Geometry: see drawing. Coordinates: mm, zero at the bounding-box minimum. A direction names the side the tool comes from. Give positions to 0.01 mm unless a question says otherwise; leave off trailing zeros. Order: outer loops, then holes, each group sorted by start corner. A loop starts at its lowest first (then second) coordinate and runs counter-clockwise, first axis right, second up. Notation, with made-up numbers: M 2,-24 L 46,-24 A21 cw 46,-11 Z; hole C 13,9.5 d7. An arc over 180 degrees is marked long. Answer as a JSON object with one key per item and string values. Group by question number.
1. Section query A-A (y = 69.85). Count the separate pieces of the cut face and the enclosed holes in it, plus the area to 3 significant figures.
2. Pull-direction query (Y, two-part tool) for the marked faces 1, 2, 3 and 4; classes: +Y half, -Y half, draft (parallel to the pull), parting line (faces both ways), or undercut.
3. Set-up query: the marked faces 5, 6, 7, 8 and 9. Return all of +Z, -Z, +X, -X, +Y, -Y with unobstructed straight access to the full face (end or side cutting, diameter ignored); none if empty.
4. Section query D-D (x = 406.5). Output: boundary loops of the cut face in (y, z), plus the area to 3 significant figures.
5. Pin query (flat end, axial travel): P1, Ø11.5, axis at x = 37.5, z = 11, coming from the +Y side; P2, Ø19, axis at y = 105.5, z = 17, coming from the -X side; P3, Ø3, axis at y = 22.5, z = 32.5, coming from the +X side; P4, Ø7.5, axis at x = 44.45, z = 19.05, coming from the -Y side. Return the tip coordinate at first contact, or that it passes through.
6. Section query C-C (x = 44.45). Output: boundary loops of the cut face in (y, z), plus the area to 3 significant figures.
7. Section query B-B (z = 19.05). Output: boundary loops of the cut face in (x, y).
8. Material intervals for L1, parallel to X at y = 71, z = 20 (1 decimal); L2, parallel to Z at x = 527, y = 81; L3, parallel to X at y = 19, z = 28.5, sorted ascending. Write a range as [from, to].
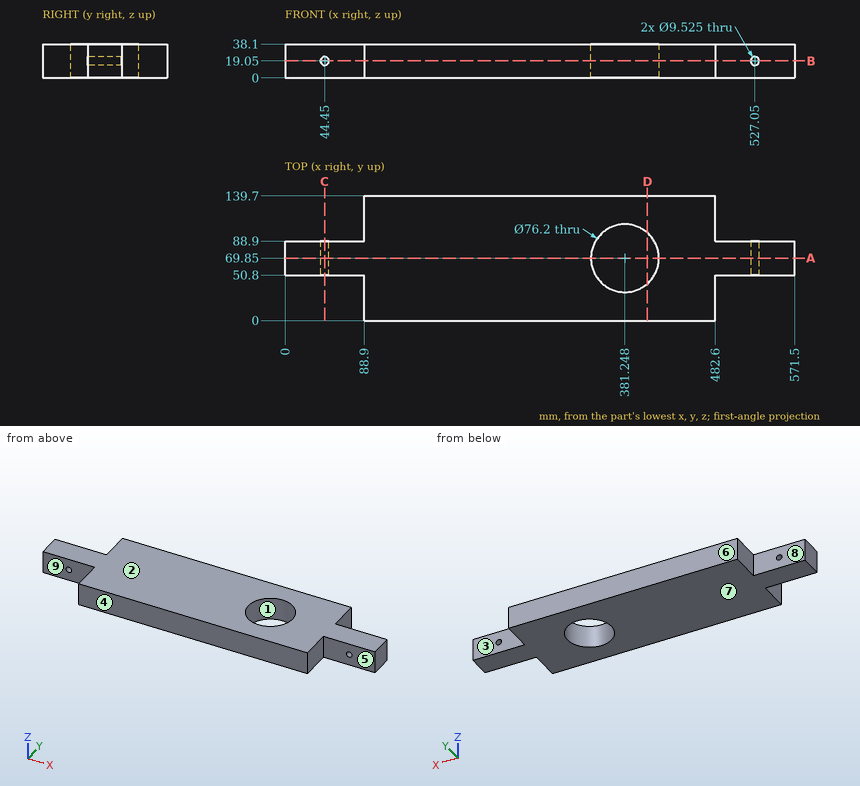
Answer sheet:
{
 "1": {"separate pieces": "2", "enclosed holes": "2", "area": "18,700 mm^2"},
 "2": {"face 1": "undercut", "face 2": "draft", "face 3": "+Y half", "face 4": "-Y half"},
 "3": {"face 5": "+Z, -Z, +X, -Y", "face 6": "+Z, -Z, +X, -X, +Y", "face 7": "-Z, +X, -X, +Y, -Y", "face 8": "+Z, -Z, -X, +Y", "face 9": "+Z, -Z, -X, -Y"},
 "4": {"outline": "M 0,0 L 41.32,0 L 41.32,38.1 L 0,38.1 Z; M 98.38,0 L 139.7,0 L 139.7,38.1 L 98.38,38.1 Z", "area": "3,150 mm^2"},
 "5": {"P1": "y = 88.9", "P2": "x = 88.9", "P3": "x = 482.6", "P4": "through"},
 "6": {"outline": "M 50.8,0 L 88.9,0 L 88.9,14.29 L 50.8,14.29 Z; M 50.8,23.81 L 88.9,23.81 L 88.9,38.1 L 50.8,38.1 Z", "area": "1,090 mm^2"},
 "7": {"outline": "M 0,50.8 L 39.69,50.8 L 39.69,88.9 L 0,88.9 Z; M 49.21,50.8 L 88.9,50.8 L 88.9,0 L 482.6,0 L 482.6,50.8 L 522.29,50.8 L 522.29,88.9 L 482.6,88.9 L 482.6,139.7 L 88.9,139.7 L 88.9,88.9 L 49.21,88.9 Z; M 531.81,50.8 L 571.5,50.8 L 571.5,88.9 L 531.81,88.9 Z; hole C 381.25,69.85 d76.2"},
 "8": {"L1": "[0, 39.8], [49.1, 343.2], [419.3, 522.4], [531.7, 571.5]", "L2": "[0, 14.29], [23.81, 38.1]", "L3": "[88.9, 482.6]"}
}
